Check sheet for the modelled part. Datum: model origin and axes. Units: mm. Face numbers are marked on the shaded views. Round coordinates to 2 decimals unless told otherwise and drop trailing zeros. Order: outer loops, then holes, each group sorted by start corner. A loop starts at its lowest first (then second) coordinate and runs counter-clockwise, first axis right, second up. Notation, with made-up numbers: (-27.75, -6.75) -> (-14.75, -6.75) arc R24 ccw to (-14.75, 14.25) -> close; hole circle Ø11 at (-32.75, 77.25). An arc over 180 degrees is marked (long way). Answer as CSV lines item,"result". Start each with the question number.
Autodesk Inventor part; units mm, degrees
ref_plane "YZ Plane" through (0, 0, 0) normal (1, 0, 0) x (0, 1, 0)
ref_plane "XZ Plane" through (0, 0, 0) normal (0, 1, 0) x (-1, 0, 0)
ref_plane "XY Plane" through (0, 0, 0) normal (0, 0, 1) x (1, 0, 0)
sketch "Sketch1" plane through (0, 0, 0) normal (0, 0, 1) x (1, 0, 0)
  line L0 (-25.4584, -1.6339) -> (-20.8864, -1.6339)
  line L1 (-20.8864, -1.6339) -> (-20.8864, -6.2059)
  line L2 (-20.8864, -6.2059) -> (-25.4584, -6.2059)
  line L3 (-25.4584, -6.2059) -> (-25.4584, -1.6339)
  line L4 (-12.7584, -6.2059) -> (-8.1864, -6.2059)
  line L5 (-8.1864, -6.2059) -> (-8.1864, -1.6339)
  line L6 (-8.1864, -1.6339) -> (-12.7584, -1.6339)
  line L7 (-12.7584, -1.6339) -> (-12.7584, -6.2059)
  line L8 (-0.0584, -6.2059) -> (4.5136, -6.2059)
  line L9 (-25.4584, 6.4941) -> (-20.8864, 6.4941)
  line L10 (-20.8864, 6.4941) -> (-20.8864, 11.0661)
  line L11 (-20.8864, 11.0661) -> (-25.4584, 11.0661)
  line L12 (-25.4584, 11.0661) -> (-25.4584, 6.4941)
  line L13 (-25.4584, 23.7661) -> (-25.4584, 19.1941)
  line L14 (-24.4424, -8.9999) -> (5.0216, -8.9999)
  line L15 (-28.2524, -5.1899) -> (-28.2524, 24.2741)
  arc A0 (-0.0584, -6.2059) -> (-25.4584, 19.1941) centre (-25.4584, -6.2059) ccw
  arc A1 (4.5136, -6.2059) -> (-25.4584, 23.7661) centre (-25.4584, -6.2059) ccw
  arc A2 (8.5693, -5.4523) -> (-24.7047, 27.8217) centre (-25.4584, -6.2059) ccw
  line L16 (-28.2524, -5.1899) -> (-24.4424, -8.9999)
  line L17 (-24.4424, -8.9999) -> (-28.2524, -5.1899)
  line L18 (-28.2524, 24.2741) -> (-24.7047, 27.8217)
  line L19 (8.5693, -5.4523) -> (5.0216, -8.9999)
  line L20 (-16.4414, 2.8111) -> (-11.8694, 2.8111)
  line L21 (-11.8694, 2.8111) -> (-11.8694, 7.3831)
  line L22 (-11.8694, 7.3831) -> (-16.4414, 7.3831)
  line L23 (-16.4414, 7.3831) -> (-16.4414, 2.8111)
  point P0 (-28.2524, -8.9999)
  point P1 (-28.2524, -8.9999)
  dimension "d0" = 4.572
  dimension "d1" = 4.572
  dimension "d2" = 4.572
  dimension "d3" = 4.572
  dimension "d4" = 4.572
  dimension "d5" = 4.572
  dimension "d6" = 8.128
  dimension "d8" = 8.128
  dimension "d10" = 4.064
  dimension "d11" = 2.794
  dimension "d12" = 2.794
  dimension "d13" = 3.81
  dimension "d14" = 3.81
  dimension "d15" = 3.81
  dimension "d16" = 3.81
  dimension "d18" = 45
  dimension "d22" = 4.572
  dimension "d23" = 4.445
  dimension "d24" = 4.445
  dimension "d25" = 4.572
extrude "Extrusion1" add sketch "Sketch1" along normal blind 0.8382
sketch "Sketch2" plane through (0, 0, 0.8382) normal (0, 0, 1) x (1, 0, 0)
  line L0 (-20.8864, -1.6339) -> (-20.8864, -6.2059)
  line L1 (-20.8864, -6.2059) -> (-25.4584, -6.2059)
  line L2 (-25.4584, -6.2059) -> (-25.4584, -1.6339)
  line L3 (-25.4584, -1.6339) -> (-20.8864, -1.6339)
  circle A0 centre (-23.1724, -3.9199) radius 2.286
  point P0 (0, 0)
surface extrude "ExtrusionSrf1" sketch "Sketch2" against normal up to surface (0.8382 mm away) shown no curves A0
pattern_linear "Rectangular Pattern1" count 2 spacing 12.7 along (1, 0, 0) of "ExtrusionSrf1"
pattern_linear "Rectangular Pattern2" count 2 spacing 12.7 along (0, 1, 0) of "ExtrusionSrf1"
sketch "Sketch3" plane through (0, 0, 0.8382) normal (0, 0, 1) x (1, 0, 0)
  line L0 (-16.4414, 2.8111) -> (-16.4414, 7.3831)
  line L1 (-16.4414, 7.3831) -> (-11.8694, 7.3831)
  line L2 (-11.8694, 7.3831) -> (-11.8694, 2.8111)
  line L3 (-11.8694, 2.8111) -> (-16.4414, 2.8111)
  circle A0 centre (-14.1554, 5.0971) radius 2.286
  point P0 (0, 0)
surface extrude "ExtrusionSrf4" sketch "Sketch3" against normal up to surface (0.8382 mm away) shown no curves A0
sketch "Sketch4" plane through (0, 0, 0.8382) normal (0, 0, 1) x (1, 0, 0)
  arc A0 (-0.0584, -6.2059) -> (-25.4584, 19.1941) centre (-25.4584, -6.2059) ccw
  line L0 (-25.4584, 19.1941) -> (-25.4584, 23.7661)
  arc A1 (4.5136, -6.2059) -> (-25.4584, 23.7661) centre (-25.4584, -6.2059) ccw
  circle A2 centre (-23.1724, 21.3855) radius 2.286
  point P0 (0, 0)
surface extrude "ExtrusionSrf5" sketch "Sketch4" against normal up to surface (0.8382 mm away) shown no curves A2
sketch "Sketch5" plane through (0, 0, 0.8382) normal (0, 0, 1) x (1, 0, 0)
  arc A0 (-0.0584, -6.2059) -> (-25.4584, 19.1941) centre (-25.4584, -6.2059) ccw
  arc A1 (4.5136, -6.2059) -> (-25.4584, 23.7661) centre (-25.4584, -6.2059) ccw
  line L0 (4.5136, -6.2059) -> (-0.0584, -6.2059)
  circle A2 centre (2.1331, -3.9199) radius 2.286
  point P0 (0, 0)
surface extrude "ExtrusionSrf6" sketch "Sketch5" against normal up to surface (0.8382 mm away) shown no curves A2
properties part number "275-1062" material "Steel"
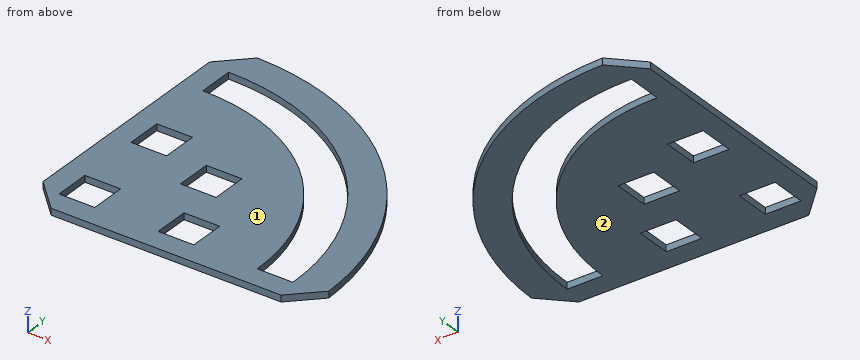
1) Section check D-D on x = -3. Record the cut outline in (y, z), then the cut area to 3 significant figures.
2) Section check A-A on y = 15.5. Record the cut outline in (x, z).
3) Material ranges on line 1 along X through (y, z) = (-4, 0.15); line 2 along Y through (x, z) = (-13.5, 0.2); line 3 along Y through (x, z) = (-25, 0.75), recorded low to high.
4) Mould release check, pull along Z, two halves, no side actions. Record for the marked faces 1 and 2: released by +Z, released by -Z, zero draft, split by the parting line, or undercut.
5) Section check B-B on x = -16. Record the cut outline in (y, z).
6) Section check C-C on z = 0.6. Record the cut outline in (x, y).
Solutions:
1,outline,"(-9, 0) -> (5.66, 0) -> (5.66, 0.84) -> (-9, 0.84) -> close; (13.64, 0) -> (19.37, 0) -> (19.37, 0.84) -> (13.64, 0.84) -> close"
1,area,"17.1 mm^2"
2,outline,"(-28.25, 0) -> (-12.27, 0) -> (-12.27, 0.84) -> (-28.25, 0.84) -> close; (-4.79, 0) -> (0.76, 0) -> (0.76, 0.84) -> (-4.79, 0.84) -> close"
3,line 1,"x = -28.25 to -25.46, -20.89 to -12.76, -8.19 to -0.15, 4.43 to 8.51"
3,line 2,"y = -9 to 2.81, 7.38 to 16.2, 21.28 to 25.66"
3,line 3,"y = -8.44 to -6.21, -1.63 to 6.49, 11.07 to 19.19, 23.76 to 27.53"
4,face 1,"released by +Z"
4,face 2,"released by -Z"
5,outline,"(-9, 0) -> (2.81, 0) -> (2.81, 0.84) -> (-9, 0.84) -> close; (7.38, 0) -> (17.37, 0) -> (17.37, 0.84) -> (7.38, 0.84) -> close; (22.23, 0) -> (26.49, 0) -> (26.49, 0.84) -> (22.23, 0.84) -> close"
6,outline,"(-28.25, -5.19) -> (-24.44, -9) -> (5.02, -9) -> (8.57, -5.45) arc R34.04 ccw to (-24.7, 27.82) -> (-28.25, 24.27) -> close; hole (-25.46, -6.21) -> (-20.89, -6.21) -> (-20.89, -1.63) -> (-25.46, -1.63) -> close; hole (-25.46, 6.49) -> (-20.89, 6.49) -> (-20.89, 11.07) -> (-25.46, 11.07) -> close; hole (-25.46, 19.19) arc R25.4 cw to (-0.06, -6.21) -> (4.51, -6.21) arc R29.97 ccw to (-25.46, 23.77) -> close; hole (-16.44, 2.81) -> (-11.87, 2.81) -> (-11.87, 7.38) -> (-16.44, 7.38) -> close; hole (-12.76, -6.21) -> (-8.19, -6.21) -> (-8.19, -1.63) -> (-12.76, -1.63) -> close"
